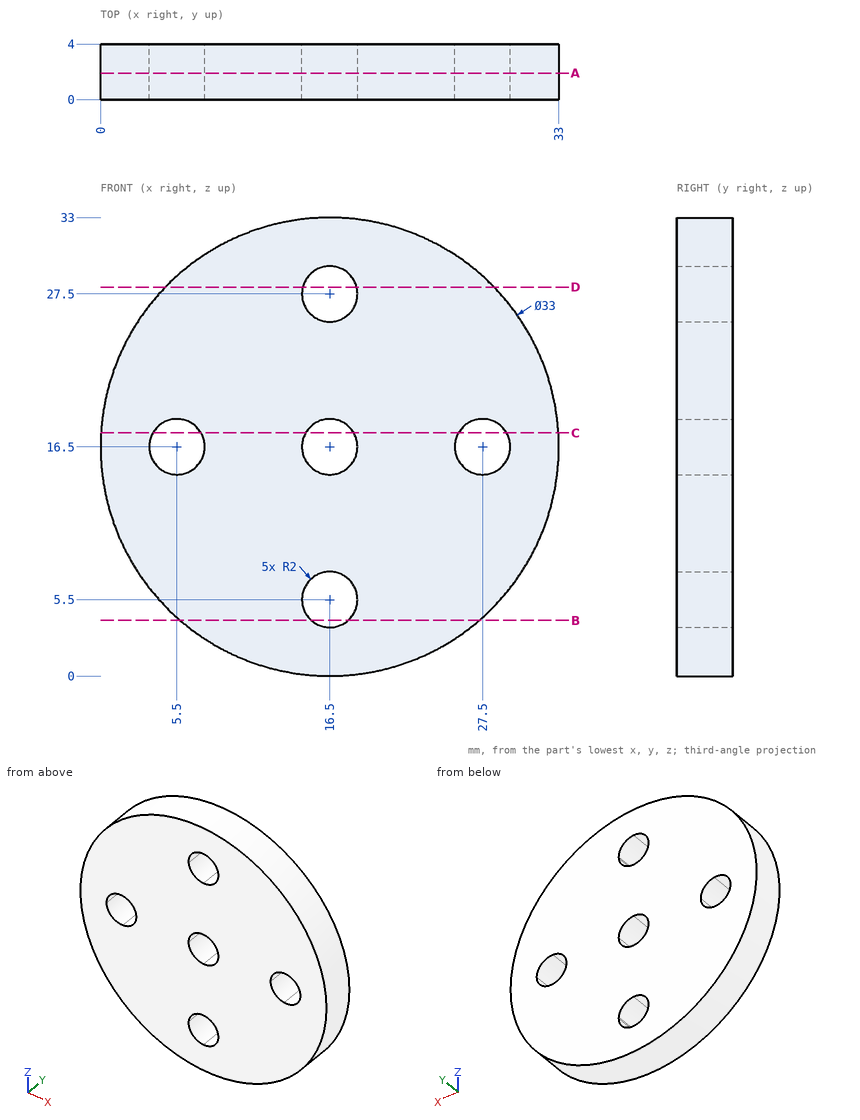
Design review of the part shown in the three views and the two pictorial views. Dimensions are in mm from the part's minimum x, y and z. Round coordinates to 2 decimals unless told otherwise and drop trailing zeros. Loops run counter-clockwise (first coordinate to the right, second up) from the corner with the lowest first, then second, coordinate; pieces in that order, holes last. Notation, with made-up numbers: M 79,-9 L 119,-9 A10 ccw 119,0 Z; hole C 1.5,4 d9. An arc over 180 degrees is marked long. Answer as a JSON object with one key per item and string values.
Item 1: Clearance check with flat-ended pins moving along their axes: P1, Ø10, axis at x = 10, z = 15, coming from the -Y side; P2, Ø2, axis at y = 1.5, z = 24, coming from the -X side; P3, Ø1.5, axis at x = 9, y = 3, coming from the +Z side; P4, Ø1.5, axis at y = 0.5, z = 8.5, coming from the +X side. State where each tip first meets the part, or that it passes through.
Check sheet entries:
{"P1": "y = 0", "P2": "x = 1.33", "P3": "z = 31.56", "P4": "x = 31.32"}
Item 2: We need section A-A, the plane y = 1.9. State the section outline as (x, z) points.
Check sheet entries:
{"outline": "C 16.5,16.5 d33; hole C 5.5,16.5 d4; hole C 16.5,5.5 d4; hole C 16.5,16.5 d4; hole C 16.5,27.5 d4; hole C 27.5,16.5 d4"}
Item 3: For line 1 along Z through (x, y) = (16, 1.2); line 2 along X through (y, z) = (1.7, 29), list the stretches that pass through material, from the lowest coordinate up.
Check sheet entries:
{"line 1": "0.01 to 3.56, 7.44 to 14.56, 18.44 to 25.56, 29.44 to 32.99", "line 2": "5.73 to 15.18, 17.82 to 27.27"}
Item 4: We need section C-C, the plane z = 17.5. State the section outline as (x, y) points, and give its area (3 significant figures).
Check sheet entries:
{"outline": "M 0.03,0 L 3.77,0 L 3.77,4 L 0.03,4 Z; M 7.23,0 L 14.77,0 L 14.77,4 L 7.23,4 Z; M 18.23,0 L 25.77,0 L 25.77,4 L 18.23,4 Z; M 29.23,0 L 32.97,0 L 32.97,4 L 29.23,4 Z", "area": "90.2 mm2"}
Item 5: We need section B-B, the plane z = 4. State the section outline as (x, y) points, and give its area (3 significant figures).
Check sheet entries:
{"outline": "M 5.73,0 L 15.18,0 L 15.18,4 L 5.73,4 Z; M 17.82,0 L 27.27,0 L 27.27,4 L 17.82,4 Z", "area": "75.6 mm2"}
Item 6: We need section D-D, the plane z = 28. State the section outline as (x, y) points.
Check sheet entries:
{"outline": "M 4.67,0 L 14.56,0 L 14.56,4 L 4.67,4 Z; M 18.44,0 L 28.33,0 L 28.33,4 L 18.44,4 Z"}
